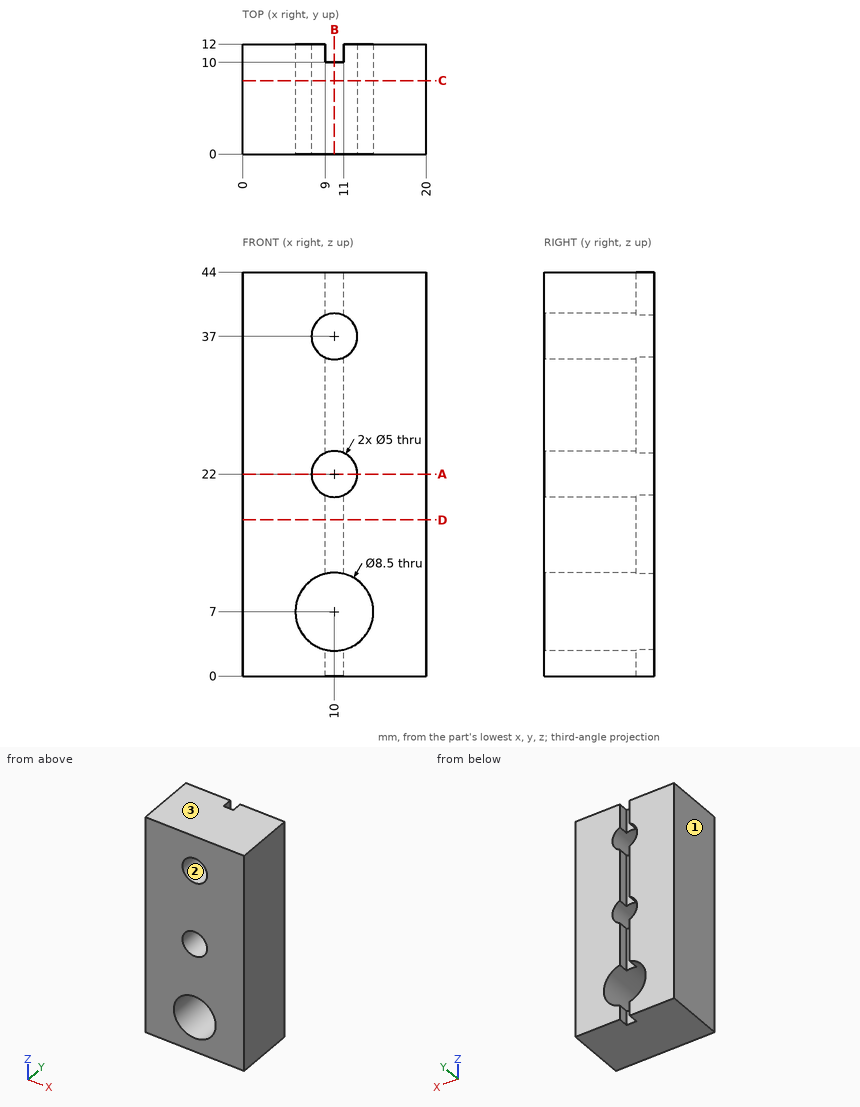
Geometry check sheet. Reference: drawing and pictorial views, mm from the part's lowest x, y, z. Coordinates: 2 decimals unless noted, no trailing zeros. Order: outer loops, then holes, each group sorted by start corner. A loop starts at its lowest first (then second) coordinate and runs counter-clockwise, first axis right, second up. Notation, with made-up numbers: (-0.75, 40) -> (35.25, 40) arc R13 ccw to (35.25, 48) -> close; hole circle Ø5 at (32, 12.5). An arc over 180 degrees is marked (long way). Write item = value, one per line. Start each with the question number.
1) Material ranges on L1, parallel to Z at x = 10, y = 2.25; L2, parallel to X at y = 10.5, z = 18; L3, parallel to X at y = 7.25, z = 22, recorded low to high.
2) Go/stop test with a flat-tipped pin: P1, Ø1.6, axis at x = 10, z = 1, coming from the +Y side. Record where the tip stops, or that it passes through.
3) Mould release check, pull along Z, two halves, no side actions. Record for the marked faces 1, 2 and 3: +Z half, -Z half, draft (parallel to the pull), parting line (faces both ways), or undercut.
4) Cross-section at D-D (z = 17). Enter the section's corners in (x, y).
5) Cross-section at A-A (z = 22). Enter the section's corners in (x, y).
6) Cross-section at C-C (y = 8). Enter the section's corners in (x, z).
7) Cross-section at B-B (x = 10). Enter the section's corners in (y, z).
Ans:
q1.L1 = 0 to 2.75, 11.25 to 19.5, 24.5 to 34.5, 39.5 to 44
q1.L2 = 0 to 9, 11 to 20
q1.L3 = 0 to 7.5, 12.5 to 20
q2.P1 = 10
q3.face_1 = draft
q3.face_2 = undercut
q3.face_3 = +Z half
q4.outline = (0, 0) -> (20, 0) -> (20, 12) -> (11, 12) -> (11, 10) -> (9, 10) -> (9, 12) -> (0, 12) -> close
q5.outline = (0, 0) -> (7.5, 0) -> (7.5, 12) -> (0, 12) -> close; (12.5, 0) -> (20, 0) -> (20, 12) -> (12.5, 12) -> close
q6.outline = (0, 0) -> (20, 0) -> (20, 44) -> (0, 44) -> close; hole circle Ø8.5 at (10, 7); hole circle Ø5 at (10, 22); hole circle Ø5 at (10, 37)
q7.outline = (0, 0) -> (10, 0) -> (10, 2.75) -> (0, 2.75) -> close; (0, 11.25) -> (10, 11.25) -> (10, 19.5) -> (0, 19.5) -> close; (0, 24.5) -> (10, 24.5) -> (10, 34.5) -> (0, 34.5) -> close; (0, 39.5) -> (10, 39.5) -> (10, 44) -> (0, 44) -> close
